Verification items for the finished model (mm, model axes). A direction names the side the tool comes from. Round coordinates to 2 decimals unless told otherwise and drop trailing zeros. Write each loop counter-clockwise with the first axis right and the second up, starting at its lowest first coordinate (ties: lowest second). Pieces come first, ordered by that corner, then holes. Notation, with made-up numbers: (-6.75, -22.75) - (16.25, -22.75) arc R19 cw to (16.25, -12.75) - close; hole circle Ø8 at (66, -38). An arc over 180 degrees is marked (long way). Answer as a JSON object with one key per item and string values.
```python
from build123d import *

# Parameters (mm, degrees)
F0_R     = 3.25
F0_W     = 100
F0_H     = 17
F0_H_2   = 5
F1_DEPTH = 5
F2_DEPTH = 15
F3_DEPTH = 60
F4_START = 55
F4_DEPTH = 5
F5_R     = 2


with BuildPart() as f1:
    # F0 (on Top) → F1 (new body)
    with BuildSketch(Plane.XY):
        Polygon((-21.7332131192, 42), (-33.5906010945, 23.5), (33.5906010945, 23.5), (21.7332131192, 42), align=None)
        with BuildLine():
            ThreePointArc((-20.5, 35), (-19.9142135624, 36.4142135624), (-18.5, 37))
            Line((-18.5, 37), (18.5, 37))
            ThreePointArc((18.5, 37), (19.9142135624, 36.4142135624), (20.5, 35))
            Line((20.5, 35), (20.5, 30.5))
            ThreePointArc((20.5, 30.5), (19.9142135624, 29.0857864376), (18.5, 28.5))
            Line((18.5, 28.5), (-18.5, 28.5))
            ThreePointArc((-18.5, 28.5), (-19.9142135624, 29.0857864376), (-20.5, 30.5))
            Line((-20.5, 30.5), (-20.5, 35))
        make_face(mode=Mode.SUBTRACT)
        Polygon((-33.5906010945, 23.5), (-40, 13.5), (40, 13.5), (33.5906010945, 23.5), align=None)
        with Locations((-20, 18.5)):
            Circle(F0_R, mode=Mode.SUBTRACT)
        with Locations((0, 18.5)):
            Circle(F0_R, mode=Mode.SUBTRACT)
        with Locations((20, 18.5)):
            Circle(F0_R, mode=Mode.SUBTRACT)
        with Locations((-20, 18.5)):
            Circle(F0_R)
        with Locations((0, 18.5)):
            Circle(F0_R)
        with Locations((20, 18.5)):
            Circle(F0_R)
        Polygon((-40, 13.5), (-50, 13.5), (-50, 8.5), (50, 8.5), (50, 13.5), (40, 13.5), align=None)
        Rectangle(F0_W, F0_H)
        with Locations((0, -11)):
            Rectangle(F0_W, F0_H_2)
    extrude(amount=F1_DEPTH)

    # F0 (on Top) → F2 (join)
    with BuildSketch(Plane.XY):
        Polygon((-33.5906010945, 23.5), (-40, 13.5), (40, 13.5), (33.5906010945, 23.5), align=None)
        with Locations((-20, 18.5)):
            Circle(F0_R, mode=Mode.SUBTRACT)
        with Locations((0, 18.5)):
            Circle(F0_R, mode=Mode.SUBTRACT)
        with Locations((20, 18.5)):
            Circle(F0_R, mode=Mode.SUBTRACT)
        Polygon((-40, 13.5), (-50, 13.5), (-50, 8.5), (50, 8.5), (50, 13.5), (40, 13.5), align=None)
        with Locations((0, -11)):
            Rectangle(F0_W, F0_H_2)
    extrude(amount=F2_DEPTH)

    # F0 (on Top) → F3 (join)
    with BuildSketch(Plane.XY):
        Polygon((-21.7332131192, 42), (-33.5906010945, 23.5), (33.5906010945, 23.5), (21.7332131192, 42), align=None)
        with BuildLine():
            ThreePointArc((-20.5, 35), (-19.9142135624, 36.4142135624), (-18.5, 37))
            Line((-18.5, 37), (18.5, 37))
            ThreePointArc((18.5, 37), (19.9142135624, 36.4142135624), (20.5, 35))
            Line((20.5, 35), (20.5, 30.5))
            ThreePointArc((20.5, 30.5), (19.9142135624, 29.0857864376), (18.5, 28.5))
            Line((18.5, 28.5), (-18.5, 28.5))
            ThreePointArc((-18.5, 28.5), (-19.9142135624, 29.0857864376), (-20.5, 30.5))
            Line((-20.5, 30.5), (-20.5, 35))
        make_face(mode=Mode.SUBTRACT)
    extrude(amount=F3_DEPTH)

    # F0 (on Top) → F4 (join)
    with BuildSketch(Plane.XY.offset(F4_START)):
        with BuildLine():
            Line((18.5, 37), (-18.5, 37))
            ThreePointArc((-18.5, 37), (-19.9142135624, 36.4142135624), (-20.5, 35))
            Line((-20.5, 35), (-20.5, 30.5))
            ThreePointArc((-20.5, 30.5), (-19.9142135624, 29.0857864376), (-18.5, 28.5))
            Line((-18.5, 28.5), (18.5, 28.5))
            ThreePointArc((18.5, 28.5), (19.9142135624, 29.0857864376), (20.5, 30.5))
            Line((20.5, 30.5), (20.5, 35))
            ThreePointArc((20.5, 35), (19.9142135624, 36.4142135624), (18.5, 37))
        make_face()
    extrude(amount=F4_DEPTH)

    # F5
    f5_edges = [f1.edges().sort_by_distance(p)[0] for p in [
        (0, 42, 0),
        (-30.866607, 27.75, 0),
        (-45, 13.5, 0),
        (-50, 0, 0),
        (0, -13.5, 0),
        (50, 0, 0),
        (45, 13.5, 0),
        (30.866607, 27.75, 0),
        (-19.914214, 36.414214, 0),
        (0, 37, 0),
        (19.914214, 36.414214, 0),
        (20.5, 32.75, 0),
        (19.914214, 29.085786, 0),
        (0, 28.5, 0),
        (-19.914214, 29.085786, 0),
        (-20.5, 32.75, 0),
        (-21.733213, 42, 30),
        (-27.661907, 32.75, 60),
        (-33.590601, 23.5, 37.5),
        (-36.795301, 18.5, 15),
        (-40, 13.5, 7.5),
        (-50, 13.5, 7.5),
        (-50, 11, 15),
        (-50, 8.5, 10),
        (-50, 0, 5),
        (-50, -8.5, 10),
        (-50, -11, 15),
        (-50, -13.5, 7.5),
        (40, 13.5, 7.5),
        (36.795301, 18.5, 15),
        (33.590601, 23.5, 37.5),
        (27.661907, 32.75, 60),
        (21.733213, 42, 30),
        (50, -13.5, 7.5),
        (50, -11, 15),
        (50, -8.5, 10),
        (50, 0, 5),
        (50, 8.5, 10),
        (50, 11, 15),
        (50, 13.5, 7.5),
        (0, 42, 60),
        (0, 23.5, 60),
        (0, -8.5, 15),
        (0, -13.5, 15),
        (0, 8.5, 15),
        (45, 13.5, 15),
        (-45, 13.5, 15),
    ]]
    fillet(f5_edges, radius=F5_R)


solid = f1.part
```
Q1. Section check A-A, the plane z = 11. State how many separate pieces and enclosed holes the cut face has, then the cut area to 3 significant figures.
Geometry check:
{"separate pieces": "2", "enclosed holes": "4", "area": "2,310 mm2"}
Q2. Set-up check for faces 5 (the cylindrical face through (-49.43, -0.15, 4.4)), 6 (the cylindrical face through (19.9, 36.43, 28.13)), 7 (the cylindrical face through (44.5, 12.9, 0.57)), 8 (the cylindrical face through (-0.423, 21.722, 9.93)), 9 (the flat face through (-1, -8.5, 9)): record each of +Z, -Z, +X, -X, +Y, -Y from which the full face is reachable in a straight line by a thin tool's end or side.
Geometry check:
{"face 5": "+Z, -X", "face 6": "-Z", "face 7": "-Z, +X, +Y", "face 8": "+Z", "face 9": "+Z, +X, -X"}
Q3. Material ranges on line 1 along Y through (x, z) = (12, 8); line 2 along Y through (x, z) = (0, 10.5); line 3 along Y through (x, z) = (43.5, 12), recorded low to high. Write a range as [from, to].
Geometry check:
{"line 1": "y = [-13.5, -8.5], [8.5, 28.5], [37, 42]", "line 2": "y = [-13.5, -8.5], [8.5, 15.25], [21.75, 28.5], [37, 42]", "line 3": "y = [-13.5, -8.5], [8.5, 13.5]"}
Q4. Section check B-B, the plane x = 0. Record the cut outline in (y, z).
Geometry check:
{"outline": "(-13.5, 2) arc R2 ccw to (-11.5, 0) - (26.5, 0) arc R2 ccw to (28.5, 2) - (28.5, 55) - (37, 55) - (37, 2) arc R2 ccw to (39, 0) - (40, 0) arc R2 ccw to (42, 2) - (42, 58) arc R2 ccw to (40, 60) - (25.5, 60) arc R2 ccw to (23.5, 58) - (23.5, 15) - (21.75, 15) - (21.75, 5) - (15.25, 5) - (15.25, 15) - (10.5, 15) arc R2 ccw to (8.5, 13) - (8.5, 5) - (-8.5, 5) - (-8.5, 13) arc R2 ccw to (-10.5, 15) - (-11.5, 15) arc R2 ccw to (-13.5, 13) - close"}
Q5. Section check D-D, the plane z = 50. Record the cut outline in (x, y), then the cut area to 3 significant figures.
Geometry check:
{"outline": "(-31.62, 26.58) arc R2 ccw to (-29.93, 23.5) - (29.93, 23.5) arc R2 ccw to (31.62, 26.58) - (22.32, 41.08) arc R2 ccw to (20.64, 42) - (-20.64, 42) arc R2 ccw to (-22.32, 41.08) - close; hole (-20.5, 30.5) arc R2 ccw to (-18.5, 28.5) - (18.5, 28.5) arc R2 ccw to (20.5, 30.5) - (20.5, 35) arc R2 ccw to (18.5, 37) - (-18.5, 37) arc R2 ccw to (-20.5, 35) - close", "area": "672 mm2"}
Q6. Section check C-C, the plane y = 1.5. Record the cut outline in (x, z), then the cut area to 3 significant figures.
Geometry check:
{"outline": "(-50, 2) arc R2 ccw to (-48, 0) - (48, 0) arc R2 ccw to (50, 2) - (50, 3) arc R2 ccw to (48, 5) - (-48, 5) arc R2 ccw to (-50, 3) - close", "area": "497 mm2"}
Q7. Gauge pin test, flat ends, axial feed: P1, Ø2, axis at x = 43, z = 10, coming from the +Y side; P2, Ø4, axis at x = 5, y = 20.5, coming from the +Z side; P3, Ø13.5, axis at x = 2.5, y = 2, coming from the +Z side. Record the tip position at first contact, or that the pin passes through.
Geometry check:
{"P1": "stops at y = 13.5", "P2": "stops at z = 15", "P3": "stops at z = 13.97"}
Q8. Release check for a two-part mould opening along Y. For faces 1 (the cylindrical face through (-49.43, -10.99, 14.4)), 2 (the cylindrical face through (-26.555, 33.42, 59.399)), 3 (the cylindrical face through (49.4, -12.93, 7.42)), 4 (the flat face through (0, 37, 28)) record: released by +Y, released by -Y, zero draft, split by the parting line, or undercut.
Geometry check:
{"face 1": "zero draft", "face 2": "released by +Y", "face 3": "released by -Y", "face 4": "undercut"}
